Can you work these out from the model? Positions are in its coordinate system, mm. Face numbers are marked on the shaded views. A direction names the side the tool comes from. Give positions to 0.01 mm unless a question says otherwise; leave off trailing zeros. Order: outer loops, then holes, each group sorted by start corner. A loop starts at its lowest first (then second) coordinate and runs counter-clockwise, first axis right, second up. Notation, with made-up numbers: (84.25, 50) - (134.25, 50) arc R10 ccw to (134.25, 62) - close; hole circle Ø3 at (44, 38). An arc over 180 degrees is marked (long way). Answer as a JSON object with one key per item and string values.
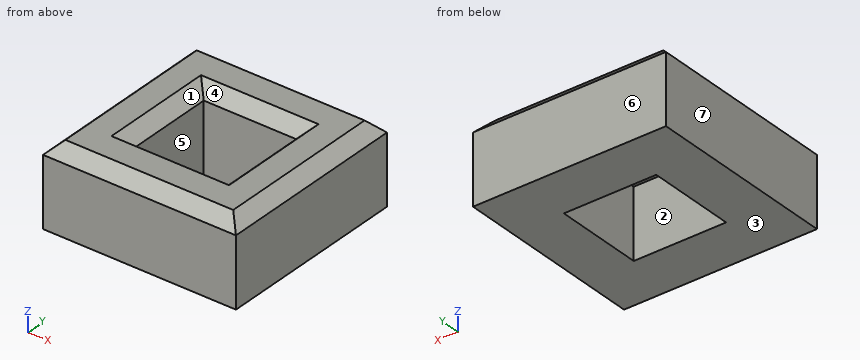
```python
from build123d import *

# Parameters (mm, degrees)
SKETCH1_W           = 15.353910524
SKETCH1_H           = 15.353910524
SKETCH1_W_2         = 7.353910524
SKETCH1_H_2         = 7.1
BOSS_EXTRUDE1_DEPTH = 6.5
CHAMFER1_SIZE       = 1


with BuildPart() as part:
    # Sketch1 → Boss-Extrude1 (new body)
    with BuildSketch(Plane.XY):
        Rectangle(SKETCH1_W, SKETCH1_H)
        Rectangle(SKETCH1_W_2, SKETCH1_H_2, mode=Mode.SUBTRACT)
    extrude(amount=BOSS_EXTRUDE1_DEPTH)

    # Chamfer1
    chamfer1_edges = [part.edges().sort_by_distance(p)[0] for p in [
        (7.676955262, 0, 6.5),
        (-3.676955262, 0, 6.5),
        (0, 7.676955262, 6.5),
        (0, -3.55, 6.5),
        (3.676955262, 0, 6.5),
        (0, 3.55, 6.5),
        (-7.676955262, 0, 6.5),
        (0, -7.676955262, 6.5),
    ]]
    chamfer(chamfer1_edges, length=CHAMFER1_SIZE)


solid = part.part
```
Q1. If we section it at C-C, the plane z = 3: Please give me the cut outline in (x, y), then the cut area to 3 significant figures.
Recorded:
{"outline": "(-7.68, -7.68) - (7.68, -7.68) - (7.68, 7.68) - (-7.68, 7.68) - close; hole (-3.68, -3.55) - (3.68, -3.55) - (3.68, 3.55) - (-3.68, 3.55) - close", "area": "184 mm^2"}
Q2. If we section it at B-B, the plane y = 0.5: Please give me the cut outline in (x, z).
Recorded:
{"outline": "(-7.68, 0) - (-3.68, 0) - (-3.68, 5.5) - (-4.68, 6.5) - (-6.68, 6.5) - (-7.68, 5.5) - close; (3.68, 0) - (7.68, 0) - (7.68, 5.5) - (6.68, 6.5) - (4.68, 6.5) - (3.68, 5.5) - close"}
Q3. I'm going to push a flat-ended pin straight in: pin 1 Ø2 at (x, y) = (4.5, 2.5) entering from +Z. Where does the tip first touch, or does it pass through?
Recorded:
{"pin 1": "stops at z = 6.5"}
Q4. We'd pull the mould along X, two halves only. Please class the marked faces 4, 5, 6 and 7: released by +X, released by -X, zero draft, split by the parting line, or undercut.
Recorded:
{"face 4": "undercut", "face 5": "undercut", "face 6": "zero draft", "face 7": "released by -X"}
Q5. If we section it at D-D, the plane y = 3.75: Please give me the cut outline in (x, z).
Recorded:
{"outline": "(-7.68, 0) - (7.68, 0) - (7.68, 5.5) - (6.68, 6.5) - (4.68, 6.5) - (3.88, 5.7) - (-3.88, 5.7) - (-4.68, 6.5) - (-6.68, 6.5) - (-7.68, 5.5) - close"}
Q6. I need wall thicknesses on L1, parallel to X at y = -1, z = 4.25; L2, parallel to Y at x = -0.25, z = 3.5. Which ranges of each line are inside material? Lowest first, please.
Recorded:
{"L1": "x = -7.68 to -3.68, 3.68 to 7.68", "L2": "y = -7.68 to -3.55, 3.55 to 7.68"}
Q7. If we section it at A-A, the plane x = 2: Please give me the cut outline in (y, z).
Recorded:
{"outline": "(-7.68, 0) - (-3.55, 0) - (-3.55, 5.5) - (-4.55, 6.5) - (-6.68, 6.5) - (-7.68, 5.5) - close; (3.55, 0) - (7.68, 0) - (7.68, 5.5) - (6.68, 6.5) - (4.55, 6.5) - (3.55, 5.5) - close"}
Q8. Which directions (+Z, -Z, +X, -X, +Y, -Y) give clear straight access to the entire face, cutting with the end or side of a thin tool? Please do the marked faces 1, 2 and 3.
Recorded:
{"face 1": "+Z", "face 2": "+Z, -Z", "face 3": "-Z, +X, -X, +Y, -Y"}
